from build123d import *

# Parameters (mm, degrees)
SKETCH_1_W          = 183.8
SKETCH_1_H          = 53.8
EXTRUDE_1_DEPTH     = 1.5
SKETCH_2_W          = 179.9
SKETCH_2_H          = 49.9
SKETCH_2_W_2        = 176.9
SKETCH_2_H_2        = 46.9
EXTRUDE_2_DEPTH     = 4
SKETCH_3_R          = 1.6
SKETCH_3_W          = 26
SKETCH_3_H          = 6
SKETCH_3_W_2        = 21
SKETCH_3_W_3        = 10.7
SKETCH_3_H_2        = 16
SKETCH_3_W_4        = 35.3
SKETCH_3_H_3        = 12.5
SKETCH_3_W_5        = 4
SKETCH_3_H_4        = 10
SKETCH_3_W_6        = 10
SKETCH_3_W_7        = 6
SKETCH_3_H_5        = 14
CUT_EXTRUDE_1_DEPTH = 10


with BuildPart() as part:
    # 草图1 → 凸台-拉伸1 (new body)
    with BuildSketch(Plane(origin=(0, 0, 0), x_dir=(1, 0, 0), z_dir=(0, 1, 0))):
        Rectangle(SKETCH_1_W, SKETCH_1_H)
    extrude(amount=EXTRUDE_1_DEPTH)

    # 草图2 → 凸台-拉伸2 (add)
    with BuildSketch(Plane(origin=(0, 1.5, 0), x_dir=(1, 0, 0), z_dir=(0, 1, 0))):
        Rectangle(SKETCH_2_W, SKETCH_2_H)
        Rectangle(SKETCH_2_W_2, SKETCH_2_H_2, mode=Mode.SUBTRACT)
    extrude(amount=EXTRUDE_2_DEPTH)

    # 草图3 → 切除-拉伸1 (cut)
    with BuildSketch(Plane.XZ):
        Circle(SKETCH_3_R)
        with Locations((-77, -10)):
            Rectangle(SKETCH_3_W, SKETCH_3_H)
        with Locations((-50.5, -10)):
            Rectangle(SKETCH_3_W_2, SKETCH_3_H)
        with Locations((-9.6, -0.35)):
            Rectangle(SKETCH_3_W_3, SKETCH_3_H_2)
        with Locations((53.3, -4.7)):
            Rectangle(SKETCH_3_W_4, SKETCH_3_H_3)
        with Locations((-31.95, 1.95)):
            Rectangle(SKETCH_3_W_5, SKETCH_3_H_4)
        with Locations((28.65, -1.45)):
            Rectangle(SKETCH_3_W_6, SKETCH_3_H)
        with Locations((-77, 2.5)):
            Rectangle(SKETCH_3_W_7, SKETCH_3_H_5)
    extrude(amount=-CUT_EXTRUDE_1_DEPTH, mode=Mode.SUBTRACT)


solid = part.part
The model under review builds one solid part; all positions refer to its coordinate system, in mm. A direction names the side the tool comes from. Give positions to 0.01 mm unless a question says otherwise; leave off trailing zeros. Loops run counter-clockwise (first coordinate to the right, second up) from the corner with the lowest first, then second, coordinate; pieces in that order, holes last. Notation, with made-up numbers: (-33.5, 76) -> (15.5, 76) arc R24 cw to (15.5, 109) -> close; hole circle Ø4 at (-20, -11). An arc over 180 degrees is marked (long way). Answer as a JSON object with one key per item and string values. Group by question number.
Q1. Take a section at D-D (x = -42). Write out the cut boundary in (y, z).
Q2. Wall thickness on line 1 along X through (y, z) = (0.9, -7.5); line 2 along Z through (x, y) = (-18.5, 1.7); line 3 along Z through (x, y) = (0, 0.85): over which ranges is each line inside the solid? List them lowest first.
Q3. Tool access review of faces 1 (the flat face through (-1, 3, -23.45)), 2 (the flat face through (-80, 1, -13)), 3 (the flat face through (-89.95, 3, 9)): name each direction out of +Z, -Z, +X, -X, +Y, -Y from which nothing blocks a thin tool from reaching the whole face with its end or side.
Q4. Insertion check: pin 1 (2 mm diameter, centred on x = -15.5, y = 3.5, fed in from -Z); pin 2 (1.5 mm diameter, centred on y = 4, z = 11.5, fed in from -X); pin 3 (1.2 mm diameter, centred on y = 3.5, z = 6.5, fed in from +X). Each pin has a flat end and moves straight along its axis. Give the tip position at first contact, or say it passes through.
Q5. Take a section at A-A (x = -12). Write out the cut boundary in (y, z).
Q6. Draft analysis for pull direction Z (two halves, no side actions). For faces 4 (the flat face through (-1, 3, 24.95)), 5 (the flat face through (89.95, 3, 0)), 6 (the flat face through (-1, 3, -24.95)), 7 (the flat face through (88.45, 3, 0)), state which applies: pulls with the +Z half, pulls with the -Z half, needs draft (parallel to the pull), parting line crosses it, or undercut.
Q7. Take a section at C-C (z = -21). Write out the cut boundary in (x, y), plus the area to 3 significant figures.
Q8. Take a section at B-B (y = 4.2). Write out the cut boundary in (x, z).
Answer below:
{
 "1": {"outline": "(0, -26.9) -> (1.5, -26.9) -> (1.5, -24.95) -> (5.5, -24.95) -> (5.5, -23.45) -> (1.5, -23.45) -> (1.5, -13) -> (0, -13) -> close; (0, -7) -> (1.5, -7) -> (1.5, 23.45) -> (5.5, 23.45) -> (5.5, 24.95) -> (1.5, 24.95) -> (1.5, 26.9) -> (0, 26.9) -> close"},
 "2": {"line 1": "x = -91.9 to -90, -64 to -61, -40 to -14.95, -4.25 to 35.65, 70.95 to 91.9", "line 2": "z = -24.95 to -23.45, 23.45 to 24.95", "line 3": "z = -26.9 to -1.6, 1.6 to 26.9"},
 "3": {"face 1": "+Y", "face 2": "+Y, -Y", "face 3": "+Z, -Z, -X, +Y"},
 "4": {"pin 1": "stops at z = -24.95", "pin 2": "stops at x = -89.95", "pin 3": "stops at x = 89.95"},
 "5": {"outline": "(0, -26.9) -> (1.5, -26.9) -> (1.5, -24.95) -> (5.5, -24.95) -> (5.5, -23.45) -> (1.5, -23.45) -> (1.5, -8.35) -> (0, -8.35) -> close; (0, 7.65) -> (1.5, 7.65) -> (1.5, 23.45) -> (5.5, 23.45) -> (5.5, 24.95) -> (1.5, 24.95) -> (1.5, 26.9) -> (0, 26.9) -> close"},
 "6": {"face 4": "pulls with the +Z half", "face 5": "needs draft", "face 6": "pulls with the -Z half", "face 7": "undercut"},
 "7": {"outline": "(-91.9, 0) -> (91.9, 0) -> (91.9, 1.5) -> (89.95, 1.5) -> (89.95, 5.5) -> (88.45, 5.5) -> (88.45, 1.5) -> (-88.45, 1.5) -> (-88.45, 5.5) -> (-89.95, 5.5) -> (-89.95, 1.5) -> (-91.9, 1.5) -> close", "area": "288 mm2"},
 "8": {"outline": "(-89.95, -24.95) -> (89.95, -24.95) -> (89.95, 24.95) -> (-89.95, 24.95) -> (-89.95, -7) -> (-88.45, -7) -> (-88.45, 23.45) -> (88.45, 23.45) -> (88.45, -23.45) -> (-88.45, -23.45) -> (-88.45, -13) -> (-89.95, -13) -> close"}
}
